Can you work these out from the model? Positions are in its coordinate system, mm. A direction names the side the tool comes from. Coordinates: 2 decimals unless noted, no trailing zeros. Order: outer loops, then holes, each group sorted by start corner. A loop starts at its lowest first (then second) coordinate and runs counter-clockwise, first axis right, second up. Notation, with made-up numbers: (-23.75, 61.25) -> (7.25, 61.25) arc R18 cw to (7.25, 95.25) -> close; hole circle Ø4 at (84, 46). An arc over 180 degrees is marked (long way). Use a Markdown table: item, result. Add a question column.
1. Suppose I cut it at C-C, the plane z = -13. List the corners of the cut face in (x, y) for me.
2. Suppose I cut it at B-B, the plane x = -31. List the corners of the cut face in (y, z) for me, then the cut area to 3 significant figures.
3. Suppose I cut it at A-A, the plane y = -5. List the corners of the cut face in (x, z) for me.
4. For faces 5 (the flat face through (10.845, -5, 5)), 6 (the cylindrical face through (10.74, -4.55, 67.68)), which set-ups out of +Z, -Z, +X, -X, +Y, -Y let a thin tool reach every point of the face, with its end or its side?
5. We'd pull the mould along X, two halves only. Please class faces 1 (the cylindrical face through (10.61, -4.55, -55.43)), 2 (the flat face through (-18, -5, 70.16)), 3 (the cylindrical face through (-48.7, 0.7, 5.4)), 4 (the cylindrical face through (9.99, -0.9, 6.97)): pulls with the +X half, pulls with the -X half, needs draft (parallel to the pull), parting line crosses it, or undercut.
6. If I drill on line 1 along Z through (x, y) = (-39, -3); line 2 along X through (y, z) = (-5, -25.5); line 3 along Y through (x, z) = (6, -45), over which ranges is the centre line in solid material (lowest first)? Write a range as from..to.
7. For pin 1 Ø4 at (y, z) = (1, 39) entering from +X; pin 2 Ø10 at (x, z) = (-11, -22) entering from -Y; pin 3 Ø2 at (y, z) = (-1, 10) entering from -X; pin 4 Ø5 at (y, z) = (-2, 8) entering from +X, each with a flat end and sliding along its axis, tell me the tip position at first contact or that it passes through.
```python
from build123d import *

# Parameters (mm, degrees)
F1_DEPTH = 6.15
F2_R     = 3
F3_T     = 2.25


with BuildPart() as f1:
    # F0 (on Front) → F1 (new body)
    with BuildSketch(Plane.XZ):
        with BuildLine():
            ThreePointArc((-41.975048, 67.910328), (-46.217689, 66.152969), (-47.975048, 61.910328))
            Line((-47.975048, 61.910328), (-47.975048, -49.529672))
            ThreePointArc((-47.975048, -49.529672), (-46.217689, -53.772313), (-41.975048, -55.529672))
            Line((-41.975048, -55.529672), (4.844952, -55.529672))
            ThreePointArc((4.844952, -55.529672), (9.087592, -53.772313), (10.844952, -49.529672))
            Line((10.844952, -49.529672), (10.844952, 61.910328))
            ThreePointArc((10.844952, 61.910328), (9.087592, 66.152969), (4.844952, 67.910328))
            Line((4.844952, 67.910328), (-41.975048, 67.910328))
        make_face()
    extrude(amount=F1_DEPTH)

    # F2
    f2_edges = [f1.edges().sort_by_distance(p)[0] for p in [
        (10.844952, 0, 6.190328),
    ]]
    fillet(f2_edges, radius=F2_R)

    # F3
    f3_openings = [f1.faces().sort_by_distance(p)[0] for p in [
        (-18.565048, -6.15, 6.190328),
    ]]
    offset(amount=F3_T, openings=f3_openings)


solid = f1.part
```
Worked out:
| question | item | result |
|---|---|---|
| 1 | outline | (-50.23, -6.15) -> (-47.98, -6.15) -> (-47.98, -3) arc R3 cw to (-44.98, 0) -> (7.84, 0) arc R3 cw to (10.84, -3) -> (10.84, -6.15) -> (13.09, -6.15) -> (13.09, -3) arc R5.25 ccw to (7.84, 2.25) -> (-44.98, 2.25) arc R5.25 ccw to (-50.23, -3) -> close |
| 2 | outline | (-6.15, -57.78) -> (-3, -57.78) arc R5.25 ccw to (2.25, -52.53) -> (2.25, 64.91) arc R5.25 ccw to (-3, 70.16) -> (-6.15, 70.16) -> (-6.15, 67.91) -> (-3, 67.91) arc R3 cw to (0, 64.91) -> (0, -52.53) arc R3 cw to (-3, -55.53) -> (-6.15, -55.53) -> close |
| 2 | area | 308 mm² |
| 3 | outline | (-50.23, -49.53) arc R8.25 ccw to (-41.98, -57.78) -> (4.84, -57.78) arc R8.25 ccw to (13.09, -49.53) -> (13.09, 61.91) arc R8.25 ccw to (4.84, 70.16) -> (-41.98, 70.16) arc R8.25 ccw to (-50.23, 61.91) -> close; hole (-47.98, -49.53) arc R6 ccw to (-41.98, -55.53) -> (4.84, -55.53) arc R6 ccw to (10.84, -49.53) -> (10.84, 61.91) arc R6 ccw to (4.84, 67.91) -> (-41.98, 67.91) arc R6 ccw to (-47.98, 61.91) -> close |
| 4 | face 5 | -Y |
| 4 | face 6 | +Z, +X, +Y, -Y |
| 5 | face 1 | pulls with the +X half |
| 5 | face 2 | needs draft |
| 5 | face 3 | pulls with the -X half |
| 5 | face 4 | undercut |
| 6 | line 1 | z = -57.78..-55.53, 67.91..70.16 |
| 6 | line 2 | x = -50.23..-47.98, 10.84..13.09 |
| 6 | line 3 | y = 0..2.25 |
| 7 | pin 1 | stops at x = 12.7 |
| 7 | pin 2 | stops at y = 0 |
| 7 | pin 3 | stops at x = -50.13 |
| 7 | pin 4 | stops at x = 13.09 |
